Geometry: final body of the model. Coordinates: model frame, mm. Give positions to 0.01 mm unless a question says otherwise; leave off trailing zeros. Order: outer loops, then holes, each group sorted by start corner. A loop starts at its lowest first (then second) coordinate and runs counter-clockwise, first axis right, second up. Notation, with made-up numbers: (66.25, 64) -> (94.25, 64) arc R15 cw to (94.25, 86) -> close; hole circle Ø10 at (-28, 60.5). An arc over 180 degrees is marked (long way). Answer in a Markdown table with one row per item. Add a question column.
Q1. Pull-direction query (X, two-part tool) for faces 1 (the face through (36.7, 21.8, 0.8)), 2 (the face through (-1, 0, 0)), 3 (the face through (-35.66, 18.35, 0.76)); classes: +X half, -X half, draft (parallel to the pull), parting line (faces both ways), or undercut.
Q2. Cut plane A-A on x = 34.35. Return the cut outline in (y, z), and give its area (3 significant figures).
Q3. Cut plane B-B on y = 19.35. Return the cut outline in (x, z), and give its area (3 significant figures).
Q4. Contact query for a flat-ended pin moving along its axis: P1, Ø5, axis at x = 11, y = 17.5, coming from the -Z side. Output: stop coordinate, or through.
Q5. Line query: line 1 along Y through (x, z) = (-34.35, 0.9); line 2 along X through (y, z) = (20, 1.4); line 3 along X through (y, z) = (-19, 1.1). Output: solid intervals per line, ascending. Write a range as from..to.
from build123d import *

# Parameters (mm, degrees)
SKETCH1_W           = 75
SKETCH1_H           = 45
BOSS_EXTRUDE1_DEPTH = 1.5
SKETCH2_R           = 1.65
CUT_EXTRUDE1_DEPTH  = 2.5


with BuildPart() as part:
    # Sketch1 → Boss-Extrude1 (new body)
    with BuildSketch(Plane.XY):
        Rectangle(SKETCH1_W, SKETCH1_H)
    extrude(amount=BOSS_EXTRUDE1_DEPTH)

    # Sketch2 → Cut-Extrude1 (cut, through all)
    with BuildSketch(Plane.XY.offset(1.5)):
        with Locations((-34.35, 19.35)):
            Circle(SKETCH2_R)
        with Locations((34.35, 19.35)):
            Circle(SKETCH2_R)
        with Locations((34.35, -19.35)):
            Circle(SKETCH2_R)
        with Locations((-34.35, -19.35)):
            Circle(SKETCH2_R)
        Polygon((-37.5, 22.5), (-36, 22.5), (-37.5, 21), align=None)
        Polygon((37.5, 22.5), (36, 22.5), (37.5, 21), align=None)
        Polygon((37.5, -21), (37.5, -22.5), (36, -22.5), align=None)
        Polygon((-37.5, -22.5), (-36, -22.5), (-37.5, -21), align=None)
    extrude(amount=-CUT_EXTRUDE1_DEPTH, mode=Mode.SUBTRACT)


solid = part.part
Completed:
| question | item | result |
|---|---|---|
| 1 | face 1 | +X half |
| 1 | face 2 | draft |
| 1 | face 3 | undercut |
| 2 | outline | (-22.5, 0) -> (-21, 0) -> (-21, 1.5) -> (-22.5, 1.5) -> close; (-17.7, 0) -> (17.7, 0) -> (17.7, 1.5) -> (-17.7, 1.5) -> close; (21, 0) -> (22.5, 0) -> (22.5, 1.5) -> (21, 1.5) -> close |
| 2 | area | 57.6 mm² |
| 3 | outline | (-37.5, 0) -> (-36, 0) -> (-36, 1.5) -> (-37.5, 1.5) -> close; (-32.7, 0) -> (32.7, 0) -> (32.7, 1.5) -> (-32.7, 1.5) -> close; (36, 0) -> (37.5, 0) -> (37.5, 1.5) -> (36, 1.5) -> close |
| 3 | area | 103 mm² |
| 4 | P1 | stops at z = 0 |
| 5 | line 1 | y = -22.5..-21, -17.7..17.7, 21..22.5 |
| 5 | line 2 | x = -37.5..-35.87, -32.83..32.83, 35.87..37.5 |
| 5 | line 3 | x = -37.5..-35.96, -32.74..32.74, 35.96..37.5 |
